Design review of the part built by this model. Coordinates are the model's own, in mm. Face numbers are marked on the shaded views. Give positions to 0.01 mm unless a question says otherwise; leave off trailing zeros. Write each loop counter-clockwise with the first axis right and the second up, starting at its lowest first coordinate (ties: lowest second). Pieces come first, ordered by that corner, then holes.
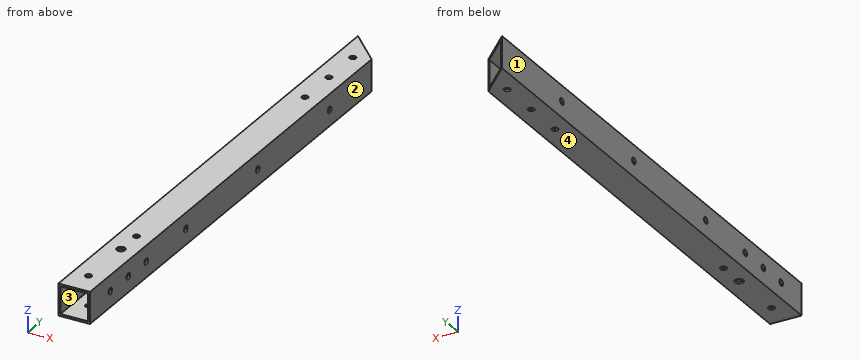
```python
from build123d import *

# Parameters (mm, degrees)
SKETCH_1_W          = 15
SKETCH_1_H          = 15
SKETCH_1_W_2        = 13
SKETCH_1_H_2        = 13
EXTRUDE_1_DEPTH     = 250
SKETCH_2_R          = 1.5
SKETCH_2_R_2        = 2
CUT_EXTRUDE_1_DEPTH = 251.561868607
SKETCH_3_R          = 1.5
CUT_EXTRUDE_2_DEPTH = 251.561868607


with BuildPart() as part:
    # 草图1 → 凸台-拉伸1 (new body)
    with BuildSketch(Plane(origin=(0, 0, 0), x_dir=(1, 0, 0), z_dir=(0, 1, 0))):
        Rectangle(SKETCH_1_W, SKETCH_1_H)
        Rectangle(SKETCH_1_W_2, SKETCH_1_H_2, mode=Mode.SUBTRACT)
    extrude(amount=EXTRUDE_1_DEPTH)

    # 草图2 → 切除-拉伸1 (cut, through all)
    with BuildSketch(Plane.XY.offset(7.5)):
        with Locations((0, 232.5)):
            Circle(SKETCH_2_R)
        with Locations((0, 212.5)):
            Circle(SKETCH_2_R)
        with Locations((0, 192.5)):
            Circle(SKETCH_2_R)
        with Locations((0, 12)):
            Circle(SKETCH_2_R)
        with Locations((0, 39)):
            Circle(SKETCH_2_R_2)
        with Locations((0, 52)):
            Circle(SKETCH_2_R)
        Polygon((7.5, 250), (7.5, 235), (-7.5, 250), align=None)
    extrude(amount=-CUT_EXTRUDE_1_DEPTH, mode=Mode.SUBTRACT)

    # 草图3 → 切除-拉伸2 (cut, through all)
    with BuildSketch(Plane(origin=(7.5, 0, 0), x_dir=(0, 0, -1), z_dir=(1, 0, 0))):
        with Locations((0, 17)):
            Circle(SKETCH_3_R)
        with Locations((0, 32)):
            Circle(SKETCH_3_R)
        with Locations((0, 47)):
            Circle(SKETCH_3_R)
        with Locations((0, 80)):
            Circle(SKETCH_3_R)
        with Locations((0, 140)):
            Circle(SKETCH_3_R)
        with Locations((0, 200)):
            Circle(SKETCH_3_R)
    extrude(amount=-CUT_EXTRUDE_2_DEPTH, mode=Mode.SUBTRACT)


solid = part.part
```
(1) Consider section A-A, the plane x = 4.25. Give the boundary of the cut face in (y, z), then the cut area to 4 significant figures.
Resolved:
outline: (0, -7.5) - (238.25, -7.5) - (238.25, -6.5) - (0, -6.5) - close; (0, 6.5) - (238.25, 6.5) - (238.25, 7.5) - (0, 7.5) - close
area: 476.5 mm2
(2) Consider section B-B, the plane z = -4. Give the boundary of the cut face in (x, y).
Resolved:
outline: (-7.5, 0) - (-6.5, 0) - (-6.5, 249) - (-7.5, 250) - close; (6.5, 0) - (7.5, 0) - (7.5, 235) - (6.5, 236) - close
(3) Mouldability with a two-part tool opening along X and no side actions: class the marked faces 1, 2, 3 and 4 as pulls with the +X half, pulls with the -X half, needs draft (parallel to the pull), parting line crosses it, or undercut.
Resolved:
face 1: pulls with the -X half
face 2: pulls with the +X half
face 3: undercut
face 4: needs draft
(4) To check wall thickness, follow L1, parallel to Z at x = -7.2, y = 80; L2, parallel to Z at x = 6, y = 62. State the ranges of each line that lie inside material, in increasing order.
Resolved:
L1: z = -7.5 to -1.5, 1.5 to 7.5
L2: z = -7.5 to -6.5, 6.5 to 7.5
(5) Clearance check with a flat-ended pin moving along its axis: P1, Ø2.5, axis at y = 17, z = 0, coming from the -X side. State where the tip first meets the part, or that it passes through.
Resolved:
P1: passes through
(6) Consider section C-C, the plane y = 180. Give the boundary of the cut face in (x, z).
Resolved:
outline: (-7.5, -7.5) - (7.5, -7.5) - (7.5, 7.5) - (-7.5, 7.5) - close; hole (-6.5, -6.5) - (6.5, -6.5) - (6.5, 6.5) - (-6.5, 6.5) - close
